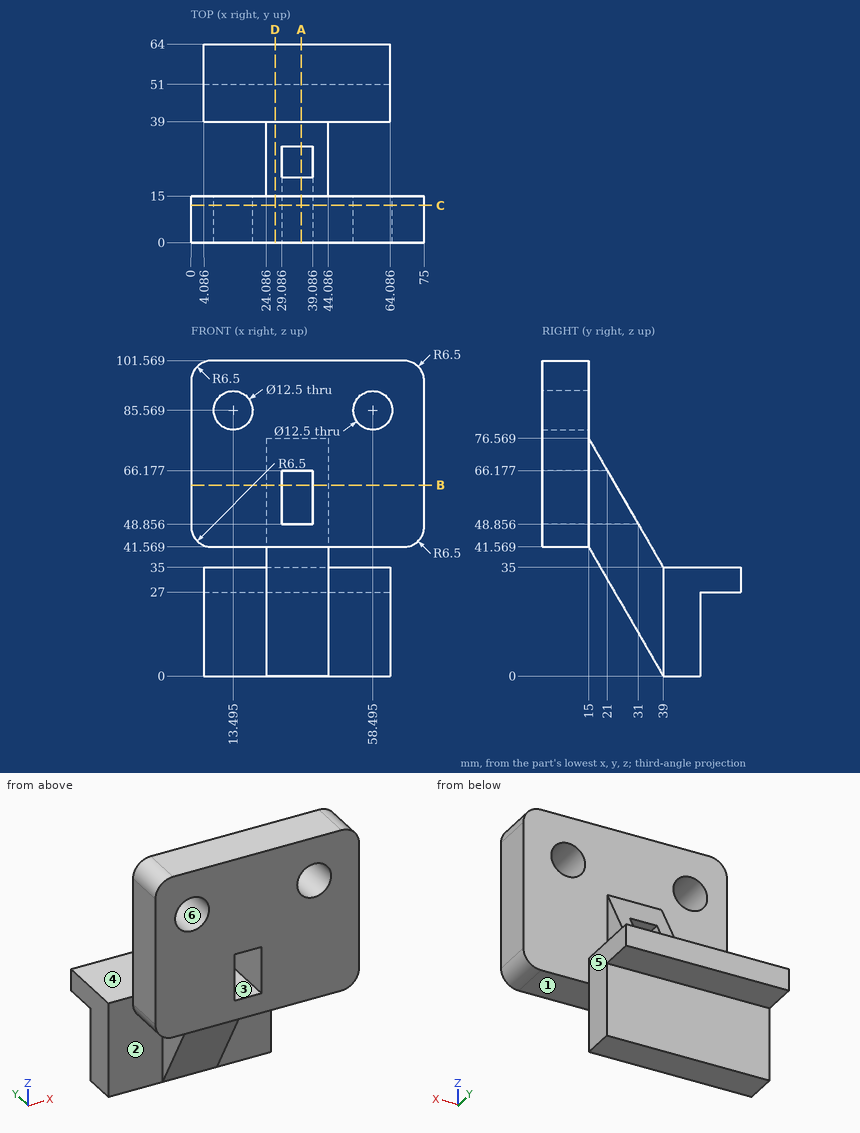
Drawing for the job (mm, zero at the part's lowest x, y, z). A direction names the side the tool comes from. Give positions to 0.01 mm unless a question says otherwise; leave off trailing zeros. Write each loop counter-clockwise with the first axis right and the second up, starting at its lowest first coordinate (ties: lowest second). Pieces come first, ordered by that corner, then holes. Notation, with made-up numbers: M 36.25,1 L 93.25,1 A25 cw 93.25,15 Z; hole C 38.25,9 d2. An arc over 180 degrees is marked long. Return JSON: item names as keys, results as strings. Group by question number.
(1) 3-axis set-ups, long thin cutter, end or side, ignore diameter. For the marked faces 1, 2 and 3: which of +Z, -Z, +X, -X, +Y, -Y reach the whole face in a straight line?
(2) Flat gauge pins, fed straight in: pin 1 Ø1.5 at (x, z) = (54.5, 58.5) entering from -Y; pin 2 Ø20 at (y, z) = (51, 17.5) entering from +X; pin 3 Ø6 at (x, z) = (59, 21.5) entering from -Y; pin 4 Ø2 at (x, y) = (27, 26.5) entering from -Z. Where does each tip first touch, or does it go through?
(3) Drill centre lines: L1, parallel to Z at x = 60.5, y = 59.5; L2, parallel to Z at x = 7, y = 5; L3, parallel to Y at x = 6.5, z = 61. Where is each one in solid material? Low to high. Write a range as [from, to].
(4) Band-saw the part on C-C (y = 12). State how many separate pieces and enclosed holes the cut face has, and give its area (4 significant figures).
(5) Band-saw the part on B-B (z = 61.5). Give the cut face in (x, y) (1 decimal).
(6) Mould opens along X. For the marked faces 4, 5 and 6 say: pulls with the +X half, pulls with the -X half, needs draft (parallel to the pull), parting line crosses it, or undercut.
(7) Band-saw the part on A-A (x = 35.5). Give the cut face in (y, z).
(8) Band-saw the part on D-D (x = 27). Give the cut face in (y, z), and give its area (3 significant figures).
Entries:
{
 "1": {"face 1": "-Z, +X, -X, -Y", "face 2": "+Z, -Z, -X, -Y", "face 3": "+Y, -Y"},
 "2": {"pin 1": "stops at y = 0", "pin 2": "stops at x = 64.09", "pin 3": "stops at y = 39", "pin 4": "stops at z = 19.92"},
 "3": {"L1": "z = [27, 35]", "L2": "z = [41.57, 101.57]", "L3": "y = [0, 15]"},
 "4": {"separate pieces": "1", "enclosed holes": "3", "area": "4,045 mm^2"},
 "5": {"outline": "M 0,0 L 29.1,0 L 29.1,23.7 L 24.1,23.7 L 24.1,15 L 0,15 Z; M 39.1,0 L 75,0 L 75,15 L 44.1,15 L 44.1,23.7 L 39.1,23.7 Z"},
 "6": {"face 4": "needs draft", "face 5": "pulls with the +X half", "face 6": "undercut"},
 "7": {"outline": "M 0,41.57 L 15,41.57 L 39,0 L 51,0 L 51,27 L 64,27 L 64,35 L 39,35 L 31,48.86 L 0,48.86 Z; M 0,66.18 L 21,66.18 L 15,76.57 L 15,101.57 L 0,101.57 Z"},
 "8": {"outline": "M 0,41.57 L 15,41.57 L 39,0 L 51,0 L 51,27 L 64,27 L 64,35 L 39,35 L 15,76.57 L 15,101.57 L 0,101.57 Z", "area": "2,260 mm^2"}
}
